Design review of the part built by this model. Coordinates are the model's own, in mm. Face numbers are marked on the shaded views. A direction names the side the tool comes from. Give positions to 0.01 mm unless a question says otherwise; leave off trailing zeros. Order: outer loops, then holes, each group sorted by start corner. A loop starts at its lowest first (then second) coordinate and runs counter-clockwise, first axis right, second up.
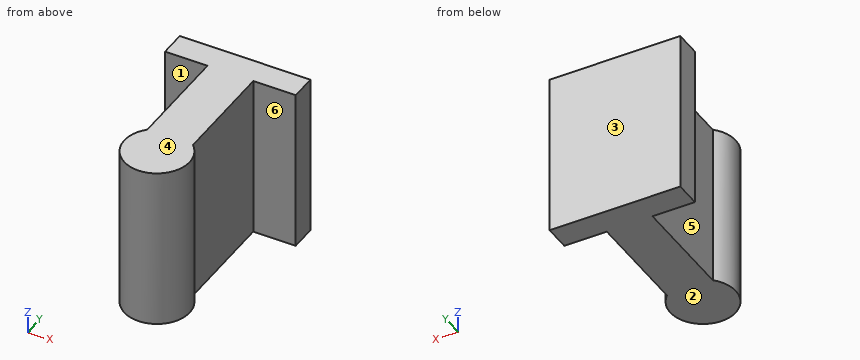
```python
from build123d import *

# Parameters (mm, degrees)
F1_DEPTH = 25


with BuildPart() as f1:
    # F0 (on Top) → F1 (new body)
    with BuildSketch(Plane.XY):
        with BuildLine():
            Line((-3.5, 20), (-3.5, 3.570714))
            ThreePointArc((-3.5, 3.570714), (0, -5), (3.5, 3.570714))
            Line((3.5, 3.570714), (3.5, 20))
            Line((3.5, 20), (10, 20))
            Line((10, 20), (10, 24))
            Line((10, 24), (-10, 24))
            Line((-10, 24), (-10, 20))
            Line((-10, 20), (-3.5, 20))
        make_face()
    extrude(amount=-F1_DEPTH)


solid = f1.part
```
1. Draft analysis for pull direction Y (two halves, no side actions). For the marked faces 1, 2 and 3, state which applies: pulls with the +Y half, pulls with the -Y half, needs draft (parallel to the pull), parting line crosses it, or undercut.
Recorded:
face 1: undercut
face 2: needs draft
face 3: pulls with the +Y half
2. Take a section at C-C (y = -3). State the section outline as (x, z) points.
Recorded:
outline: (-4, -25) - (4, -25) - (4, 0) - (-4, 0) - close
3. Take a section at A-A (z = -7). State the section outline as (x, y) points, then the cut area to 3 significant figures.
Recorded:
outline: (-10, 20) - (-3.5, 20) - (-3.5, 3.57) arc R5 ccw (long way) to (3.5, 3.57) - (3.5, 20) - (10, 20) - (10, 24) - (-10, 24) - close
area: 267 mm2
4. For pin 1 (3 mm diameter, centred on x = 7.5, z = -10.5, fed in from -Y); pin 2 (8 mm diameter, centred on y = 8, z = -16, fed in from +X); pin 3 (5 mm diameter, centred on x = -7, y = 16.5, fed in from +Z); pin 4 (5 mm diameter, centred on y = 13.5, z = -9.5, fed in from -X), all flat-tipped, find the tip position at first contact; note any pin that passes through.
Recorded:
pin 1: stops at y = 20
pin 2: stops at x = 3.5
pin 3: passes through
pin 4: stops at x = -3.5
5. Take a section at B-B (y = 0). State the section outline as (x, z) points.
Recorded:
outline: (-5, -25) - (5, -25) - (5, 0) - (-5, 0) - close
6. For line 1 along Y through (x, z) = (9, -13); line 2 along X through (y, z) = (17.5, -5.5); line 3 along Y through (x, z) = (-2.75, -20.75), list the stretches that pass through material, from the lowest coordinate up.
Recorded:
line 1: y = 20 to 24
line 2: x = -3.5 to 3.5
line 3: y = -4.18 to 24
7. Machinability: for the marked faces 4, 5 and 6, which of the approach directions +Z, -Z, +X, -X, +Y, -Y give a long, thin tool a straight path to every point of the face, cutting with its end or side? Answer none if there is none.
Recorded:
face 4: +Z, +X, -X, +Y, -Y
face 5: +Z, -Z, -X
face 6: +Z, -Z, +X
